Build history of the part. All positions in model axes, mm. Face numbers are marked on the shaded views. A direction names the side the tool comes from. Round coordinates to 2 decimals unless told otherwise and drop trailing zeros. Write each loop counter-clockwise with the first axis right and the second up, starting at its lowest first coordinate (ties: lowest second). Pieces come first, ordered by that corner, then holes. Notation, with made-up numbers: (75.25, 46) -> (99.25, 46) arc R15 cw to (99.25, 63) -> close; hole circle Ø8 at (5.5, -38.5). An arc over 180 degrees is marked (long way). Answer as CSV lines item,"result".
from build123d import *

# Parameters (mm, degrees)
F0_W     = 25.4
F0_H     = 25.4
F0_W_2   = 22.225
F0_H_2   = 22.225
F1_DEPTH = 25.4
F2_DEPTH = 23.8125
F3_R     = 3.175
F4_DEPTH = 3.175


with BuildPart() as f1:
    # F0 (on Top) → F1 (new body)
    with BuildSketch(Plane.XY):
        with Locations((0, 12.7)):
            Rectangle(F0_W, F0_H)
        with Locations((0, 12.7)):
            Rectangle(F0_W_2, F0_H_2, mode=Mode.SUBTRACT)
        with Locations((0, 12.7)):
            Rectangle(F0_W_2, F0_H_2)
    extrude(amount=F1_DEPTH)

    # F0 (on Top) → F2 (cut)
    with BuildSketch(Plane.XY):
        with Locations((0, 12.7)):
            Rectangle(F0_W_2, F0_H_2)
    extrude(amount=F2_DEPTH, mode=Mode.SUBTRACT)

    # F3 (on face) → F4 (join)
    with BuildSketch(Plane.XY.offset(25.4)):
        with Locations((7.9375, 4.7625)):
            Circle(F3_R)
        with Locations((7.9375, 20.6375)):
            Circle(F3_R)
        with Locations((-7.9375, 20.6375)):
            Circle(F3_R)
        with Locations((-7.9375, 4.7625)):
            Circle(F3_R)
    extrude(amount=F4_DEPTH)


solid = f1.part
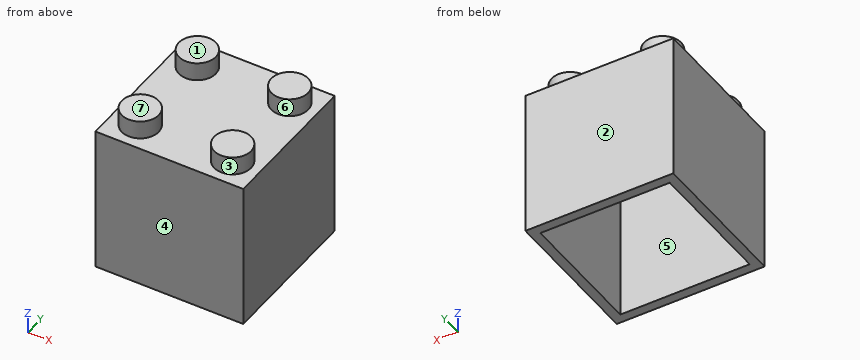
1. Drop a flat-ended pin along its axis: pin 1 Ø7.5 at (x, y) = (2, 14.5) entering from +Z. Give the stop position or say it passes through.
Results found:
pin 1,"stops at z = 25.4"
2. Probe line 1 along X through (y, z) = (18.25, 23.5); line 2 along Y through (x, z) = (6.5, 23.25); line 3 along Z through (x, y) = (9.25, 15.5). List the from-to ranges inside material, lowest first.
Results found:
line 1,"x = -12.7 to -11.11, 11.11 to 12.7"
line 2,"y = 0 to 1.59, 23.81 to 25.4"
line 3,"z = 23.81 to 25.4"
3. Mould opens along Y. For the marked faces 1, 2, 3 and 4 say: +Y half, -Y half, draft (parallel to the pull), parting line (faces both ways), or undercut.
Results found:
face 1,"draft"
face 2,"+Y half"
face 3,"undercut"
face 4,"-Y half"
4. Which spindle directions (+Z, -Z, +X, -X, +Y, -Y) get a long thin tool onto all of the face, cutting with end or side? Do the marked faces 5, 6 and 7. Say none if no direction does.
Results found:
face 5,"-Z"
face 6,"+Z"
face 7,"+Z, +X, -X, +Y, -Y"
5. Cut at C-C, the plane y = 14.25. Write the cut outline in (x, z).
Results found:
outline,"(-12.7, 0) -> (-11.11, 0) -> (-11.11, 23.81) -> (11.11, 23.81) -> (11.11, 0) -> (12.7, 0) -> (12.7, 25.4) -> (-12.7, 25.4) -> close"
6. Cut at A-A, the plane z = 9.75. Write the cut outline in (x, y), then the cut area to 3 significant figures.
Results found:
outline,"(-12.7, 0) -> (12.7, 0) -> (12.7, 25.4) -> (-12.7, 25.4) -> close; hole (-11.11, 1.59) -> (11.11, 1.59) -> (11.11, 23.81) -> (-11.11, 23.81) -> close"
area,"151 mm2"
7. Cut at B-B, the plane x = 0.25. Write the cut outline in (y, z).
Results found:
outline,"(0, 0) -> (1.59, 0) -> (1.59, 23.81) -> (23.81, 23.81) -> (23.81, 0) -> (25.4, 0) -> (25.4, 25.4) -> (0, 25.4) -> close"
8. Cut at D-D, the plane x = 7.5. Write the cut outline in (y, z) (1 decimal), then the cut area to 3 significant figures.
Results found:
outline,"(0, 0) -> (1.6, 0) -> (1.6, 23.8) -> (23.8, 23.8) -> (23.8, 0) -> (25.4, 0) -> (25.4, 25.4) -> (23.8, 25.4) -> (23.8, 28.6) -> (17.5, 28.6) -> (17.5, 25.4) -> (7.9, 25.4) -> (7.9, 28.6) -> (1.6, 28.6) -> (1.6, 25.4) -> (0, 25.4) -> close"
area,"156 mm2"
